from build123d import *

# Parameters (mm, degrees)
SKETCH1_R               = 4.95
SKETCH1_W               = 17.9
SKETCH1_H               = 45.1
BOSS_EXTRUDE1_DEPTH     = 3.5
CUT_EXTRUDE1_DEPTH      = 251.796682357
CUT_EXTRUDE1_DEPTH_BACK = 251.796682357
SKETCH2_W               = 258.160615752
SKETCH2_H               = 10
SKETCH3_W               = 12
SKETCH3_H               = 60
BOSS_EXTRUDE2_DEPTH     = 3.5
FILLET1_R               = 20
BOSS_EXTRUDE3_START     = -3.5
BOSS_EXTRUDE3_DEPTH     = 3.5
CIRPATTERN1_COUNT       = 9
SKETCH5_W               = 17
SKETCH5_H               = 3.5
CUT_EXTRUDE2_DEPTH      = 250.910895112
CUT_EXTRUDE3_DEPTH      = 250.910895112


with BuildPart() as part:
    # Sketch1 → Boss-Extrude1 (new body)
    with BuildSketch(Plane.YZ):
        with BuildLine():
            Line((-10.899695646, -10.305175148), (-129.080307876, -215))
            Line((-129.080307876, -215), (-88.665789032, -215))
            Line((-88.665789032, -215), (-17.790269987, -92.24))
            Line((-17.790269987, -92.24), (17.790269987, -92.24))
            Line((17.790269987, -92.24), (88.665789032, -215))
            Line((88.665789032, -215), (129.080307876, -215))
            Line((129.080307876, -215), (10.899695646, -10.305175148))
            ThreePointArc((10.899695646, -10.305175148), (0, 15), (-10.899695646, -10.305175148))
        make_face()
        with Locations(Location((0, 0, 0), (0, 0, 270))):
            Circle(SKETCH1_R, mode=Mode.SUBTRACT)
        with Locations((0, -54.69)):
            Rectangle(SKETCH1_W, SKETCH1_H, mode=Mode.SUBTRACT)
    extrude(amount=BOSS_EXTRUDE1_DEPTH)

    # Sketch2 → Cut-Extrude1 (cut, two sides: drawn at the far end of the back side and taken through both)
    with BuildSketch(Plane.YZ.offset(3.5).offset(-CUT_EXTRUDE1_DEPTH_BACK)):
        with Locations((0, -210)):
            Rectangle(SKETCH2_W, SKETCH2_H)
    extrude(amount=CUT_EXTRUDE1_DEPTH + CUT_EXTRUDE1_DEPTH_BACK, mode=Mode.SUBTRACT)

    # Sketch3 → Boss-Extrude2 (add)
    with BuildSketch(Plane(origin=(3.5, 0, 0), x_dir=(0, 0, -1), z_dir=(1, 0, 0))):
        with Locations((199, -112.892286341)):
            Rectangle(SKETCH3_W, SKETCH3_H)
        with Locations((199, 112.892286341)):
            Rectangle(SKETCH3_W, SKETCH3_H)
    extrude(amount=-BOSS_EXTRUDE2_DEPTH)

    # Fillet1
    fillet1_edges = [part.edges().sort_by_distance(p)[0] for p in [
        (1.75, -116.378601954, -193),
        (1.75, 116.378601954, -193),
    ]]
    fillet(fillet1_edges, radius=FILLET1_R)

    # Sketch4 → Boss-Extrude3 (add)
    with BuildSketch(Plane(origin=(3.5, 0, 0), x_dir=(0, 0, -1), z_dir=(1, 0, 0)).offset(BOSS_EXTRUDE3_START)):
        with BuildLine():
            Line((-14.095389312, 5.13030215), (-34.137962787, 0))
            Line((-34.137962787, 0), (-15, 0))
            ThreePointArc((-15, 0), (-14.772116295, 2.604722665), (-14.095389312, 5.13030215))
        make_face()
        with BuildLine():
            Line((-34.137962787, 0), (-14.095389312, -5.13030215))
            ThreePointArc((-14.095389312, -5.13030215), (-14.772116295, -2.604722665), (-15, 0))
            Line((-15, 0), (-34.137962787, 0))
        make_face()
    boss_extrude3 = extrude(amount=BOSS_EXTRUDE3_DEPTH)

    # CirPattern1: Boss-Extrude3 ×9 about axis
    cirpattern1_axis = Axis((0, 0, 0), (1, 0, 0))
    for i in range(1, CIRPATTERN1_COUNT):
        add(boss_extrude3.rotate(cirpattern1_axis, i * 360 / CIRPATTERN1_COUNT))

    # Sketch5 → Cut-Extrude2 (cut, symmetric)
    with BuildSketch(Plane(origin=(3.5, 0, 0), x_dir=(0, 0, -1), z_dir=(1, 0, 0))):
        with Locations((191.5, -126.142286341)):
            Rectangle(SKETCH5_W, SKETCH5_H)
    cut_extrude2 = extrude(amount=CUT_EXTRUDE2_DEPTH, both=True, mode=Mode.SUBTRACT)

    # Mirror1: Cut-Extrude2 across plane
    add(cut_extrude2.mirror(Plane.ZX), mode=Mode.SUBTRACT)

    # Sketch6 → Cut-Extrude3 (cut, symmetric)
    with BuildSketch(Plane.YZ.offset(3.5)):
        Polygon((-15.413378072, -72.19421526), (-14.95, -71.844331927), (-14.95, -32.59506202), (-19.146348264, -44.729209649), (-33.320603167, -85.715441185), (-16.757760632, -73.209319511), align=None)
        Polygon((-40.452020015, -87.978847078), (-27.957868434, -51.850797102), (-58.475794969, -104.709396402), (-41.912952433, -92.203274728), align=None)
        Polygon((-44.440620352, -126.565865893), (-18.81339339, -82.279763058), (-34.966746745, -94.476691336), (-36.374058239, -98.54606889), align=None)
        Polygon((-53.243788825, -135.456403713), (-43.245914121, -100.728050325), (-59.700544534, -113.152464165), (-68.824966717, -146.420983438), align=None)
        Polygon((-80.442842118, -188.780872527), (-54.234238638, -143.490099921), (-68.345208144, -153.420084111), (-71.318419935, -155.512353255), align=None)
        Polygon((-76.978433226, -153.464848336), (-68.249306861, -121.637615567), (-99.099637478, -175.071955626), (-80.672732205, -157.159147315), align=None)
        Polygon((-112.914500338, -199), (-89.467175046, -199), (-88.913955872, -196.982909779), (-80.146284863, -165.015139537), (-102.228944471, -186.481709354), (-110.110561046, -194.143434684), align=None)
    cut_extrude3 = extrude(amount=CUT_EXTRUDE3_DEPTH, both=True, mode=Mode.SUBTRACT)

    # Mirror2: Cut-Extrude3 across plane
    add(cut_extrude3.mirror(Plane.ZX), mode=Mode.SUBTRACT)


solid = part.part
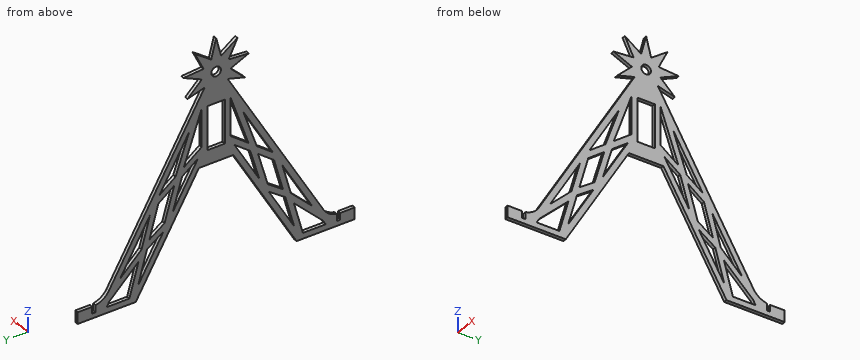
Geometry check sheet. Reference: the model listing, model coordinates, mm. Give positions to 0.01 mm unless a question says otherwise; leave off trailing zeros. Answer in a Markdown table with one row per item. Add a question column.
1) Material ranges on probe 1 along Y at (x, z) = (1.6, -56.5); probe 2 along Y at (x, z) = (3.1, -34); probe 3 along Z at (x, y) = (1.45, 13.5), recorded low to high. Write a range as from..to.
2) Gauge pin test, flat ends, axial feed: P1, Ø1.8, axis at x = 2, z = -62.5, coming from the +Y side; P2, Ø1.8, axis at x = 1.5, y = 136, coming from the +Z side; P3, Ø1.8, axis at x = 1, y = -4.5, coming from the -Z side; P4, Ø9, axis at y = 0, z = 0, coming from the +X side. Record the tip position at first contact, or that the pin passes through.
3) Cross-section at A-A on x = 1.15. State how many separate pieces and enclosed holes the cut face has, and give its area (3 significant figures).
Outcome:
| question | item | result |
|---|---|---|
| 1 | probe 1 | y = -37.57..-30.64, -29.57..-23.22, -14.95..-8.95, 8.95..14.95, 23.22..29.57, 30.64..37.57 |
| 1 | probe 2 | y = -24.58..-15.44, -14.95..-8.95, 8.95..14.95, 15.44..24.58 |
| 1 | probe 3 | z = -92.24..-14.81, -12.57..7.46, 8.56..20.1 |
| 2 | P1 | stops at y = 41.55 |
| 2 | P2 | stops at z = -193 |
| 2 | P3 | stops at z = -92.24 |
| 2 | P4 | passes through |
| 3 | separate pieces | 1 |
| 3 | enclosed holes | 16 |
| 3 | area | 11,400 mm^2 |
